The listing builds one solid part. Answer for the finished solid, in the listing's coordinates (mm). Face numbers are marked on the shaded views. Give positions to 0.01 mm unless a question says otherwise; leave off trailing zeros. Write each loop counter-clockwise with the first axis right and the second up, starting at its lowest first coordinate (ties: lowest second). Pieces come first, ordered by that corner, then holes. Notation, with made-up numbers: M -4,-22 L 50,-22 A21 cw 50,-12 Z; hole C 75.25,16.5 d4. An arc over 180 degrees is marked long. Return JSON: item names as keys, results as strings.
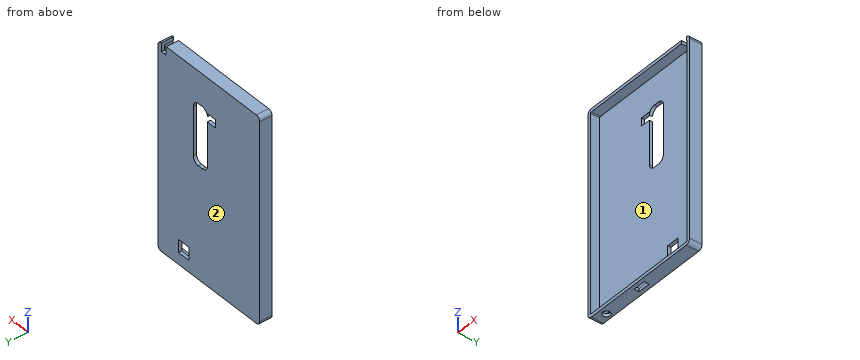
from build123d import *

# Parameters (mm, degrees)
F1_DEPTH = 7.5438
F4_T     = -2
F3_W     = 7.7331361671
F3_H     = 7.36
F3_W_2   = 3.617387048
F3_H_2   = 5.1309723878
F3_W_3   = 7.83
F3_H_3   = 7.83
F5_DEPTH = 50.8
F6_DEPTH = 25.4
F7_DEPTH = 50.8
F2_R     = 2.2388813648
F2_W     = 7.5641849544
F2_H     = 3.0062778387
F8_DEPTH = 2


with BuildPart() as f1:
    # F0 (on Front) → F1 (new body)
    with BuildSketch(Plane.XZ):
        with BuildLine():
            Line((37.6971361852, 55.4623973095), (-33.0543925679, 55.4623973095))
            ThreePointArc((-33.0543925679, 55.4623973095), (-34.8504437921, 54.7184485338), (-35.5943925679, 52.9223973095))
            Line((-35.5943925679, 52.9223973095), (-35.5943925679, -66.9464466786))
            ThreePointArc((-35.5943925679, -66.9464466786), (-34.8504437921, -68.7424979029), (-33.0543925679, -69.4864466786))
            Line((-33.0543925679, -69.4864466786), (37.6971361852, -69.4864466786))
            ThreePointArc((37.6971361852, -69.4864466786), (39.4931874094, -68.7424979029), (40.2371361852, -66.9464466786))
            Line((40.2371361852, -66.9464466786), (40.2371361852, 52.9223973095))
            ThreePointArc((40.2371361852, 52.9223973095), (39.4931874094, 54.7184485338), (37.6971361852, 55.4623973095))
        make_face()
    extrude(amount=-F1_DEPTH)

    # F4
    f4_openings = [f1.faces().sort_by_distance(p)[0] for p in [
        (2.321372, 0, -7.012025),
    ]]
    offset(amount=F4_T, openings=f4_openings)

    # F3 (on face) → F5 (cut)
    with BuildSketch(Plane(origin=(0, 7.5438, 0), x_dir=(-1, 0, 0), z_dir=(0, 1, 0))):
        with BuildLine():
            Line((-7.1636471725, 35.889052581), (-10.0967833396, 35.889052581))
            ThreePointArc((-10.0967833396, 35.889052581), (-12.7908601759, 34.7731294173), (-13.9067833396, 32.079052581))
            Line((-13.9067833396, 32.079052581), (-13.9067833396, 22.249052581))
            Line((-13.9067833396, 22.249052581), (-3.3536471725, 22.249052581))
            Line((-3.3536471725, 22.249052581), (-3.3536471725, 29.0738900152))
            Line((-3.3536471725, 29.0738900152), (-3.3536471725, 32.079052581))
            ThreePointArc((-3.3536471725, 32.079052581), (-4.4695703362, 34.7731294173), (-7.1636471725, 35.889052581))
        make_face()
        Polygon((-3.3536471725, 34.0338900152), (-3.3536471725, 32.079052581), (-3.3536471725, 29.0738900152), (2.4879228336, 29.0738900152), (2.4879228336, 34.0338900152), align=None)
        with BuildLine():
            Line((-3.3536471725, 22.249052581), (-13.9067833396, 22.249052581))
            Line((-13.9067833396, 22.249052581), (-13.9067833396, 2.459052581))
            ThreePointArc((-13.9067833396, 2.459052581), (-12.7908601759, -0.2350242554), (-10.0967833396, -1.350947419))
            Line((-10.0967833396, -1.350947419), (-7.1636471725, -1.350947419))
            ThreePointArc((-7.1636471725, -1.350947419), (-4.4695703362, -0.2350242554), (-3.3536471725, 2.459052581))
            Line((-3.3536471725, 2.459052581), (-3.3536471725, 22.249052581))
        make_face()
        with Locations((-8.630215256, 10.449052581)):
            Rectangle(F3_W, F3_H, mode=Mode.SUBTRACT)
        with Locations((-35.8884426612, 52.8969111156)):
            Rectangle(F3_W_2, F3_H_2)
        with Locations((-21.0011794782, -58.4082461512)):
            Rectangle(F3_W_3, F3_H_3)
    extrude(amount=-F5_DEPTH, mode=Mode.SUBTRACT)

    # F6 (add): a face of the model
    f6_faces = [f1.faces().sort_by_distance(p)[0] for p in [
        (8.630215256, 7.5438, 10.449052581),
    ]]
    extrude(f6_faces, amount=F6_DEPTH)

    # F7 (cut): a face of the model
    f7_faces = [f1.faces().sort_by_distance(p)[0] for p in [
        (8.630215256, 32.9438, 10.449052581),
    ]]
    extrude(f7_faces, amount=-F7_DEPTH, mode=Mode.SUBTRACT)

    # F2 (on face) → F8 (cut)
    with BuildSketch(Plane(origin=(0, 0, -69.4864466786), x_dir=(1, 0, 0), z_dir=(0, 0, -1))):
        with Locations((-26.7510712147, -4.0631839074)):
            Circle(F2_R)
        with Locations((-0.0824703602, -3.7237651413)):
            Rectangle(F2_W, F2_H)
    extrude(amount=-F8_DEPTH, mode=Mode.SUBTRACT)


solid = f1.part
Item 1: Determine the mould class of the marked faces 1 and 2 for opening direction Z: +Z half, -Z half, draft (parallel to the pull), parting line (faces both ways), or undercut.
Geometry results:
{"face 1": "undercut", "face 2": "draft"}
Item 2: A cutting plane is placed at B-B, the plane x = -22.5. Write down the section's boundary in (y, z), plus the area to 3 significant figures.
Geometry results:
{"outline": "M 0,-69.49 L 7.54,-69.49 L 7.54,55.46 L 0,55.46 L 0,53.46 L 5.54,53.46 L 5.54,-67.49 L 0,-67.49 Z", "area": "272 mm2"}
Item 3: A cutting plane is placed at A-A, the plane z = 25. Write down the section's boundary in (x, y), plus the area to 3 significant figures.
Geometry results:
{"outline": "M -35.59,0 L -33.59,0 L -33.59,5.54 L 3.35,5.54 L 3.35,7.54 L -35.59,7.54 Z; M 13.91,5.54 L 38.24,5.54 L 38.24,0 L 40.24,0 L 40.24,7.54 L 13.91,7.54 Z", "area": "153 mm2"}
Item 4: A cutting plane is placed at C-C, the plane z = -3. Write down the section's boundary in (x, y), plus the area to 3 significant figures.
Geometry results:
{"outline": "M -35.59,0 L -33.59,0 L -33.59,5.54 L 38.24,5.54 L 38.24,0 L 40.24,0 L 40.24,7.54 L -35.59,7.54 Z", "area": "174 mm2"}
Item 5: Find the intervals of material crossed by line 1 (Z direction, x = -5, y = 2); line 2 (X direction, y = 4, z = 18.5); line 3 (Y direction, x = 20, z = -27.5), in increasing order.
Geometry results:
{"line 1": "z = -69.49 to -67.49, 53.46 to 55.46", "line 2": "x = -35.59 to -33.59, 38.24 to 40.24", "line 3": "y = 5.54 to 7.54"}
Item 6: Given pin 1 Ø1.6 at (y, z) = (4, -68) entering from -X, flat-ended and moving along its own axis, determine where the tip first touches the part or whether it passes through.
Geometry results:
{"pin 1": "stops at x = -35.58"}
Item 7: A cutting plane is placed at D-D, the plane x = 35.5. Write down the section's boundary in (y, z), plus the area to 3 significant figures.
Geometry results:
{"outline": "M 0,-69.49 L 7.54,-69.49 L 7.54,50.33 L 5.54,50.33 L 5.54,-67.49 L 0,-67.49 Z", "area": "251 mm2"}
